from build123d import *

# Parameters (mm, degrees)
SKETCH1_W           = 2.5
SKETCH1_H           = 25
SKETCH2_W           = 6.130760382
SKETCH2_H           = 11
BOSS_EXTRUDE1_DEPTH = 25
CIRPATTERN1_COUNT   = 5
SKETCH3_W           = 6.130760382
SKETCH3_H           = 12
BOSS_EXTRUDE2_DEPTH = 25
CIRPATTERN2_COUNT   = 5


with BuildPart() as part:
    # Sketch1 → Revolve1 (revolve)
    with BuildSketch(Plane(origin=(0, 0, 0), x_dir=(0, 0, -1), z_dir=(1, 0, 0))):
        with Locations((21.25, 49.5)):
            Rectangle(SKETCH1_W, SKETCH1_H)
        with Locations((21.25, 12.5)):
            Rectangle(SKETCH1_W, SKETCH1_H)
        Polygon((5, 25), (5, 0), (10, 0), (10, 25), (10, 37), (10, 62), (5, 62), (5, 37), align=None)
        Polygon((5, 25), (5, 0), (10, 0), (10, 25), (10, 37), (10, 62), (5, 62), (5, 37), align=None)
    revolve(axis=Axis((0, 0, 0), (0, 1, 0)))

    # Sketch2 → Boss-Extrude1 (add)
    with BuildSketch(Plane.XZ):
        with Locations((0, 15.018584153)):
            Rectangle(SKETCH2_W, SKETCH2_H)
    boss_extrude1 = extrude(amount=-BOSS_EXTRUDE1_DEPTH)

    # CirPattern1: Boss-Extrude1 ×5 about axis
    cirpattern1_axis = Axis((0, 0, 0), (0, 1, 0))
    for i in range(1, CIRPATTERN1_COUNT):
        add(boss_extrude1.rotate(cirpattern1_axis, i * 360 / CIRPATTERN1_COUNT))

    # Sketch3 → Boss-Extrude2 (add)
    with BuildSketch(Plane(origin=(0, 62, 0), x_dir=(-1, 0, 0), z_dir=(0, 1, 0))):
        with Locations((0, 14.863932977)):
            Rectangle(SKETCH3_W, SKETCH3_H)
    boss_extrude2 = extrude(amount=-BOSS_EXTRUDE2_DEPTH)

    # CirPattern2: Boss-Extrude2 ×5 about axis
    cirpattern2_axis = Axis((0, 0, 0), (0, 1, 0))
    for i in range(1, CIRPATTERN2_COUNT):
        add(boss_extrude2.rotate(cirpattern2_axis, i * 360 / CIRPATTERN2_COUNT))


solid = part.part
For this review, take the finished solid that the model builds, in its own axes (mm). A direction names the side the tool comes from. Round coordinates to 2 decimals unless told otherwise and drop trailing zeros. Loops run counter-clockwise (first coordinate to the right, second up) from the corner with the lowest first, then second, coordinate; pieces in that order, holes last. Notation, with made-up numbers: (25, -4) - (37, -4) arc R36 ccw to (37, 31) - close; hole circle Ø5 at (38.25, -16). An arc over 180 degrees is marked (long way). Use one line per item in the form item = value.
1) We need section D-D on x = 12. Write out the cut boundary in (y, z).
Solutions:
outline = (0, -19.03) - (25, -19.03) - (25, -11.3) - (0, -11.3) - close; (0, 0.68) - (25, 0.68) - (25, 7.12) - (0, 7.12) - close; (0, 16) - (25, 16) - (25, 19.03) - (0, 19.03) - close; (37, -19.03) - (62, -19.03) - (62, -11.3) - (37, -11.3) - close; (37, 0.68) - (62, 0.68) - (62, 7.12) - (37, 7.12) - close; (37, 16) - (62, 16) - (62, 19.03) - (37, 19.03) - close
2) Mouldability with a two-part tool opening along X and no side actions: class faces 3 (the face through (-2, 0, -5)), 4 (the face through (-12.909, 49.675, 7.418)) as pulls with the +X half, pulls with the -X half, needs draft (parallel to the pull), parting line crosses it, or undercut.
Solutions:
face_3 = needs draft
face_4 = undercut
3) Wall thickness on probe 1 along X at (y, z) = (42, 0); probe 2 along Z at (x, y) = (0, 47); probe 3 along Z at (x, y) = (0, 31.5): over which ranges is each line inside the solid? List them lowest first.
Solutions:
probe_1 = -22.5 to -20, -10 to -5, 5 to 10, 20 to 22.5
probe_2 = -22.5 to -20, -10 to -5, 5 to 22.5
probe_3 = -10 to -5, 5 to 10
4) We need section A-A on y = 13.5. Write out the cut boundary in (x, z).
Solutions:
outline = circle Ø45 at (0, 0); hole (-19.74, 3.19) arc R20 ccw to (-14.1, -14.19) - (-8.07, -5.9) arc R10 cw to (-10, 0.03) - close; hole (-17.85, 9.02) - (-8.11, 5.86) arc R10 cw to (-3.07, 9.52) - (-3.07, 19.76) arc R20 ccw to start; hole (-9.14, -17.79) arc R20 ccw to (9.14, -17.79) - (3.11, -9.5) arc R10 cw to (-3.11, -9.5) - close; hole circle Ø10 at (0, 0); hole (3.07, 9.52) arc R10 cw to (8.11, 5.86) - (17.85, 9.02) arc R20 ccw to (3.07, 19.76) - close; hole (8.07, -5.9) - (14.1, -14.19) arc R20 ccw to (19.74, 3.19) - (10, 0.03) arc R10 cw to start
5) We need section C-C on z = -8. Write out the cut boundary in (x, y).
Solutions:
outline = (-21.03, 0) - (-18.33, 0) - (-18.33, 25) - (-21.03, 25) - close; (-21.03, 37) - (-18.33, 37) - (-18.33, 62) - (-21.03, 62) - close; (-9.6, 0) - (9.6, 0) - (9.6, 25) - (6, 25) - (6, 37) - (9.6, 37) - (9.6, 62) - (-9.6, 62) - (-9.6, 37) - (-6, 37) - (-6, 25) - (-9.6, 25) - close; (18.33, 0) - (21.03, 0) - (21.03, 25) - (18.33, 25) - close; (18.33, 37) - (21.03, 37) - (21.03, 62) - (18.33, 62) - close
6) Tool access review of faces 1 (the face through (-12.909, 12.325, 7.418)), 2 (the face through (11, 25, 1)): name each direction out of +Z, -Z, +X, -X, +Y, -Y from which nothing blocks a thin tool from reaching the whole face with its end or side.
Solutions:
face_1 = +Y, -Y
face_2 = none
7) We need section B-B on x = 0. Write out the cut boundary in (y, z), then the cut area to 3 significant figures.
Solutions:
outline = (0, -22.5) - (25, -22.5) - (25, -20) - (0, -20) - close; (0, -10) - (62, -10) - (62, -5) - (0, -5) - close; (0, 5) - (62, 5) - (62, 22.5) - (37, 22.5) - (37, 10) - (25, 10) - (25, 22.5) - (0, 22.5) - close; (37, -22.5) - (62, -22.5) - (62, -20) - (37, -20) - close
area = 1,370 mm2
8) Clearance check with flat-ended pins moving along their axes: P1, Ø4, axis at x = 14.5, z = -1, coming from the +Y side; P2, Ø5, axis at y = 30, z = -8.5, coming from the -X side; P3, Ø3, axis at y = 51, z = 12, coming from the -X side; P4, Ø10, axis at y = 34, z = -7.5, coming from the +X side. State where each tip first meets the part, or that it passes through.
Solutions:
P1 = through
P2 = -8
P3 = -19.9
P4 = 22.23
